Here's how the part is built. I have some questions about the finished solid (model axes, mm). A direction names the side the tool comes from. Round coordinates to 2 decimals unless told otherwise and drop trailing zeros. Write each loop counter-clockwise with the first axis right and the second up, starting at its lowest first coordinate (ties: lowest second). Pieces come first, ordered by that corner, then holes. Notation, with made-up numbers: (-21, -31) -> (13, -31) arc R18 cw to (13, -24) -> close; hole circle Ø7 at (-7.75, -8.5). An arc over 180 degrees is marked (long way). Answer in a Markdown table with one row per item.
from build123d import *

# Parameters (mm, degrees)
SKETCH_4_R          = 2.5
SKETCH_4_W          = 21
SKETCH_4_H          = 40.1
EXTRUDE_1_DEPTH     = 4
SKETCH_5_W          = 5.5
SKETCH_5_H          = 5.5
CUT_EXTRUDE_5_DEPTH = 10
FILLET_1_R          = 5
SKETCH_6_R          = 3
CUT_EXTRUDE_6_DEPTH = 2


with BuildPart() as part:
    # 草图4 → 凸台-拉伸1 (new body)
    with BuildSketch(Plane.XY):
        Polygon((-30.514243596, -31.085830111), (-0.514243596, -31.085830111), (-0.514243596, 43.914169889), (-30.514243596, 43.914169889), (-45.514243596, 43.914169889), (-45.514243596, -31.085830111), align=None)
        with Locations((-22.614243596, 24.699169889)):
            Circle(SKETCH_4_R, mode=Mode.SUBTRACT)
        with Locations((-12.614243596, 24.699169889)):
            Circle(SKETCH_4_R, mode=Mode.SUBTRACT)
        with Locations((-12.614243596, -24.800830111)):
            Circle(SKETCH_4_R, mode=Mode.SUBTRACT)
        with Locations((-22.614243596, -24.800830111)):
            Circle(SKETCH_4_R, mode=Mode.SUBTRACT)
        with Locations((-17.614243596, -0.000830111)):
            Rectangle(SKETCH_4_W, SKETCH_4_H, mode=Mode.SUBTRACT)
    extrude(amount=EXTRUDE_1_DEPTH)

    # 草图5 → 切除-拉伸5 (cut)
    with BuildSketch(Plane(origin=(0, 0, 0), x_dir=(-1, 0, 0), z_dir=(0, 0, -1))):
        Polygon((42.514243596, 3.414169889), (42.514243596, 6.414169889), (42.514243596, 8.914169889), (37.014243596, 8.914169889), (37.014243596, 3.414169889), align=None)
        with Locations((39.764243596, 29.414169889)):
            Rectangle(SKETCH_5_W, SKETCH_5_H)
        with Locations((39.764243596, -16.585830111)):
            Rectangle(SKETCH_5_W, SKETCH_5_H)
    extrude(amount=-CUT_EXTRUDE_5_DEPTH, mode=Mode.SUBTRACT)

    # 圆角1
    fillet_1_edges = [part.edges().sort_by_distance(p)[0] for p in [
        (-45.514243596, -31.085830111, 2),
        (-45.514243596, 43.914169889, 2),
        (-0.514243596, 43.914169889, 2),
        (-0.514243596, -31.085830111, 2),
    ]]
    fillet(fillet_1_edges, radius=FILLET_1_R)

    # 草图6 → 切除-拉伸6 (cut)
    with BuildSketch(Plane(origin=(0, 0, 0), x_dir=(-1, 0, 0), z_dir=(0, 0, -1))):
        with Locations((17.614243596, 25.504169889)):
            Circle(SKETCH_6_R)
    extrude(amount=-CUT_EXTRUDE_6_DEPTH, mode=Mode.SUBTRACT)


solid = part.part
1) I want a section at A-A, the plane x = -27. List the corners of the cut face in (y, z) for me.
Response:
| item | result |
|---|---|
| outline | (-31.09, 0) -> (-20.05, 0) -> (-20.05, 4) -> (-31.09, 4) -> close; (20.05, 0) -> (43.91, 0) -> (43.91, 4) -> (20.05, 4) -> close |
2) I want a section at C-C, the plane y = -12. List the corners of the cut face in (x, z) for me.
Response:
| item | result |
|---|---|
| outline | (-45.51, 0) -> (-28.11, 0) -> (-28.11, 4) -> (-45.51, 4) -> close; (-7.11, 0) -> (-0.51, 0) -> (-0.51, 4) -> (-7.11, 4) -> close |
3) I need wall thicknesses on line 1 (X direction, y = -25, z = 3.7); line 2 (X direction, y = -4.5, z = 1.1); line 3 (Y direction, x = -26, z = 3.7). Which ranges of each line are inside material? Lowest first, please. Write a range as [from, to].
Response:
| item | result |
|---|---|
| line 1 | x = [-45.51, -25.11], [-20.12, -15.11], [-10.12, -0.51] |
| line 2 | x = [-45.51, -28.11], [-7.11, -0.51] |
| line 3 | y = [-31.09, -20.05], [20.05, 43.91] |
4) I want a section at B-B, the plane y = 8. List the corners of the cut face in (x, z) for me.
Response:
| item | result |
|---|---|
| outline | (-45.51, 0) -> (-42.51, 0) -> (-42.51, 4) -> (-45.51, 4) -> close; (-37.01, 0) -> (-28.11, 0) -> (-28.11, 4) -> (-37.01, 4) -> close; (-7.11, 0) -> (-0.51, 0) -> (-0.51, 4) -> (-7.11, 4) -> close |
5) I want a section at D-D, the plane z = 2.7. Count the separate pieces of the cut face and the enclosed holes in it, and give its area (3 significant figures).
Response:
| item | result |
|---|---|
| separate pieces | 1 |
| enclosed holes | 8 |
| area | 2,340 mm^2 |
6) Which directions (+Z, -Z, +X, -X, +Y, -Y) give clear straight access to the entire face, cutting with the end or side of a thin tool? Please do faces 1 (the face through (-42.514, 6, 2)), 2 (the face through (-44.01, -29.66, 2.03)), 3 (the face through (-17.57, 22.504, 0.986)).
Response:
| item | result |
|---|---|
| face 1 | +Z, -Z |
| face 2 | +Z, -Z, -X, -Y |
| face 3 | -Z |
